CAD build for the part. Positions are in the model's coordinates, mm. A direction names the side the tool comes from. Round coordinates to 2 decimals unless told otherwise and drop trailing zeros. Loops run counter-clockwise (first coordinate to the right, second up) from the corner with the lowest first, then second, coordinate; pieces in that order, holes last. Notation, with made-up numbers: M 76.5,29.25 L 103.5,29.25 A17 ccw 103.5,49.25 Z; hole C -16.75,84.5 d11. An arc over 180 degrees is marked long. Use a Markdown table: item, result. Add a question column.
(1) Band-saw the part on D-D, the plane x = 2. Write the cut outline in (y, z).
(2) Two-plate mould, pull along X, no slides. Class faces 4 (the face through (-23.49, 10.89, 3.45)), 5 (the face through (-10, -12.7, 3)), 6 (the face through (-16, 8.89, 3)): released by +X, released by -X, zero draft, split by the parting line, or undercut.
(3) Wall check: L1, parallel to X at y = -5.5, z = 6; L2, parallel to X at y = 0, z = 5.9; L3, parallel to Y at x = -18, z = 4. Give the ranges that are in metal, low to high.
(4) Band-saw the part on B-B, the plane x = -14. Write the cut outline in (y, z).
(5) Band-saw the part on A-A, the plane y = 0. Write the cut outline in (x, z), and give its area (3 significant figures).
(6) Band-saw the part on C-C, the plane z = 6.5. Write the cut outline in (x, y), and give its area (3 significant figures).
(7) Which spindle directions (+Z, -Z, +X, -X, +Y, -Y) get a long thin tool onto all of the face, cutting with end or side? Do faces 1 (the face through (-1.73, -7.81, 4.46)), 2 (the face through (12.697, -0.279, 3.451)), 3 (the face through (-21.59, 6.29, 3.45)). Say none if no direction does.
from build123d import *

# Parameters (mm, degrees)
F0_R     = 8
F1_DEPTH = 7
F2_R     = 8
F2_R_2   = 5
F3_DEPTH = 2


with BuildPart() as f1:
    # F0 (on Top) → F1 (new body)
    with BuildSketch(Plane.XY):
        with BuildLine():
            ThreePointArc((0, -12.7), (12.7, 0), (0, 12.7))
            Line((0, 12.7), (-19.05, 12.7))
            ThreePointArc((-19.05, 12.7), (-23.540128, 10.840128), (-25.4, 6.35))
            Line((-25.4, 6.35), (-25.4, -6.35))
            ThreePointArc((-25.4, -6.35), (-23.540128, -10.840128), (-19.05, -12.7))
            Line((-19.05, -12.7), (0, -12.7))
        make_face()
        with BuildLine():
            Line((-12.7, -8.89), (-19.05, -8.89))
            ThreePointArc((-19.05, -8.89), (-21.59, -6.35), (-19.05, -3.81))
            Line((-19.05, -3.81), (-12.7, -3.81))
            ThreePointArc((-12.7, -3.81), (-10.16, -6.35), (-12.7, -8.89))
        make_face(mode=Mode.SUBTRACT)
        Circle(F0_R, mode=Mode.SUBTRACT)
        with BuildLine():
            Line((-12.7, 3.81), (-19.05, 3.81))
            ThreePointArc((-19.05, 3.81), (-21.59, 6.35), (-19.05, 8.89))
            Line((-19.05, 8.89), (-12.7, 8.89))
            ThreePointArc((-12.7, 8.89), (-10.16, 6.35), (-12.7, 3.81))
        make_face(mode=Mode.SUBTRACT)
    extrude(amount=F1_DEPTH)

    # F2 (on face) → F3 (join)
    with BuildSketch(Plane(origin=(0, 0, 0), x_dir=(1, 0, 0), z_dir=(0, 0, -1))):
        Circle(F2_R)
        Circle(F2_R_2, mode=Mode.SUBTRACT)
    extrude(amount=-F3_DEPTH)


solid = f1.part
Return value:
| question | item | result |
|---|---|---|
| 1 | outline | M -12.54,0 L -4.58,0 L -4.58,2 L -7.75,2 L -7.75,7 L -12.54,7 Z; M 4.58,0 L 12.54,0 L 12.54,7 L 7.75,7 L 7.75,2 L 4.58,2 Z |
| 2 | face 4 | released by -X |
| 2 | face 5 | zero draft |
| 2 | face 6 | undercut |
| 3 | L1 | -25.4 to -21.44, -10.31 to -5.81, 5.81 to 11.45 |
| 3 | L2 | -25.4 to -8, 8 to 12.7 |
| 3 | L3 | -12.7 to -8.89, -3.81 to 3.81, 8.89 to 12.7 |
| 4 | outline | M -12.7,0 L -8.89,0 L -8.89,7 L -12.7,7 Z; M -3.81,0 L 3.81,0 L 3.81,7 L -3.81,7 Z; M 8.89,0 L 12.7,0 L 12.7,7 L 8.89,7 Z |
| 5 | outline | M -25.4,0 L -5,0 L -5,2 L -8,2 L -8,7 L -25.4,7 Z; M 5,0 L 12.7,0 L 12.7,7 L 8,7 L 8,2 L 5,2 Z |
| 5 | area | 167 mm^2 |
| 6 | outline | M -25.4,-6.35 A6.35 ccw -19.05,-12.7 L 0,-12.7 A12.7 ccw 0,12.7 L -19.05,12.7 A6.35 ccw -25.4,6.35 Z; hole M -19.05,-8.89 L -12.7,-8.89 A2.54 ccw -12.7,-3.81 L -19.05,-3.81 A2.54 ccw Z; hole M -19.05,3.81 L -12.7,3.81 A2.54 ccw -12.7,8.89 L -19.05,8.89 A2.54 ccw Z; hole C 0,0 d16 |
| 6 | area | 575 mm^2 |
| 7 | face 1 | +Z |
| 7 | face 2 | +Z, -Z, +X |
| 7 | face 3 | +Z, -Z |
